```python
from build123d import *

# Parameters (mm, degrees)
F1_DEPTH      = 2
F2_DEPTH      = 42
F5_DEPTH      = 2
F7_DEPTH      = 2
F8_W          = 28.9586056024
F8_H          = 21
F9_DEPTH      = 25
F10_W         = 38.9921951145
F10_H         = 12
F11_DEPTH     = 2
F12_T1_DEPTH  = 12
F12_T6_DEPTH  = 51.7431402671
F12_T11_DEPTH = 51.7431402671
F12_T17_DEPTH = 40
F12_T22_DEPTH = 51.7431402671
F13_R         = 5


# Not quite as in the source:
# - a fillet or chamfer that OpenCascade refuses, or shapes differently, is made with other operations: its cross-section is extruded or revolved along the edge and cut away or added


with BuildPart() as f1:
    # F0 (on Top) → F1 (new body)
    with BuildSketch(Plane.XY):
        Polygon((16.9007111498, 56.5512960928), (-61.0992888502, 51.6762960928), (-61.0992888502, 18.6762960928), (16.9007111498, 13.8012960928), (18.9007111498, 13.6762960928), (18.9007111498, 15.6801985355), (16.9007111498, 15.8051985355), (-59.0992888502, 20.5551985355), (-59.0992888502, 49.79739365), (16.9007111498, 54.54739365), (18.9007111498, 54.67239365), (18.9007111498, 56.6762960928), align=None)
        Polygon((18.9007111498, 15.6801985355), (18.9007111498, 54.67239365), (16.9007111498, 54.54739365), (16.9007111498, 15.8051985355), align=None)
        Polygon((16.9007111498, 15.8051985355), (16.9007111498, 54.54739365), (-59.0992888502, 49.79739365), (-59.0992888502, 20.5551985355), align=None)
    extrude(amount=F1_DEPTH)

    # F0 (on Top) → F2 (join)
    with BuildSketch(Plane.XY):
        Polygon((16.9007111498, 56.5512960928), (-61.0992888502, 51.6762960928), (-61.0992888502, 18.6762960928), (16.9007111498, 13.8012960928), (18.9007111498, 13.6762960928), (18.9007111498, 15.6801985355), (16.9007111498, 15.8051985355), (-59.0992888502, 20.5551985355), (-59.0992888502, 49.79739365), (16.9007111498, 54.54739365), (18.9007111498, 54.67239365), (18.9007111498, 56.6762960928), align=None)
    extrude(amount=F2_DEPTH)

    # F3 (on face) → F5 (join)
    with BuildSketch(Plane(origin=(0.9249861815, 14.7997789033, 0), x_dir=(0.9980525785, -0.0623782862, 0), z_dir=(-0.0623782862, -0.9980525785, 0))):
        Polygon((18.3653086424, 55), (-62.1452981224, 42), (18.010799587, 42), align=None)
    extrude(amount=-F5_DEPTH)

    # F6 (on face) → F7 (join)
    with BuildSketch(Plane(origin=(-3.4549417367, 55.2790677874, 0), x_dir=(-0.9980525785, -0.0623782862, 0), z_dir=(-0.0623782862, 0.9980525785, 0))):
        Polygon((-22.3992737141, 55), (-22.3992737141, 42), (57.7568239953, 42), align=None)
    extrude(amount=-F7_DEPTH)

    # F8 (on face) → F9 (cut)
    with BuildSketch(Plane(origin=(-61.0992888502, 0, 0), x_dir=(0, -1, 0), z_dir=(-1, 0, 0))):
        with Locations((-35.0762708113, 31.5)):
            Rectangle(F8_W, F8_H)
    extrude(amount=-F9_DEPTH, mode=Mode.SUBTRACT)

    # F10 (on face) → F11 (join)
    with BuildSketch(Plane.YZ.offset(18.9007111498)):
        with Locations((35.1762960928, 21)):
            Rectangle(F10_W, F10_H)
    extrude(amount=-F11_DEPTH)

    # F12: fillet of radius 5 on 4 edges, made by hand

    # F12_s2 → F12_t1 (join)
    with BuildSketch(Plane.XY.offset(15)):
        with BuildLine():
            ThreePointArc((11.588819719, 16.1371917499), (15.324199345, 17.4833184516), (16.9007111498, 21.1274546423))
            Line((16.9007111498, 21.1274546423), (16.9007111498, 15.8051985355))
            Line((16.9007111498, 15.8051985355), (11.588819719, 16.1371917499))
        make_face()
        with BuildLine():
            ThreePointArc((11.588819719, 54.2154004356), (15.324199345, 52.869273734), (16.9007111498, 49.2251375432))
            Line((16.9007111498, 49.2251375432), (16.9007111498, 54.54739365))
            Line((16.9007111498, 54.54739365), (11.588819719, 54.2154004356))
        make_face()
    extrude(amount=F12_T1_DEPTH)


with BuildPart() as f12_tool4:
    # F12_s5 → F12_t6 (new body)
    with BuildSketch(Plane.XY.offset(2)):
        with BuildLine():
            ThreePointArc((-54.411180281, 20.2621917499), (-57.743425041, 21.8289664471), (-59.0992888502, 25.2524546423))
            Line((-59.0992888502, 25.2524546423), (-59.0992888502, 20.5551985355))
            Line((-59.0992888502, 20.5551985355), (-54.411180281, 20.2621917499))
        make_face()
    extrude(amount=F12_T6_DEPTH)

    split(bisect_by=Plane.XY.offset(21), keep=Keep.BOTTOM)


with BuildPart() as f1_1:
    add(f1.part)

    # F12_t3: union F12_tool4
    add(f12_tool4.part)


with BuildPart() as f12_tool9:
    # F12_s10 → F12_t11 (new body)
    with BuildSketch(Plane.XY.offset(-9.7431402671)):
        with BuildLine():
            ThreePointArc((-54.411180281, 20.2621917499), (-57.743425041, 21.8289664471), (-59.0992888502, 25.2524546423))
            Line((-59.0992888502, 25.2524546423), (-59.0992888502, 20.5551985355))
            Line((-59.0992888502, 20.5551985355), (-54.411180281, 20.2621917499))
        make_face()
    extrude(amount=F12_T11_DEPTH)

    split(bisect_by=Plane.XZ.offset(-20.5969680101), keep=Keep.TOP)

    split(bisect_by=Plane.XY.offset(21), keep=Keep.TOP)


with BuildPart() as f1_2:
    add(f1_1.part)

    # F12_t8: union F12_tool9
    add(f12_tool9.part)


with BuildPart() as f12_tool15:
    # F12_s16 → F12_t17 (new body)
    with BuildSketch(Plane.XY.offset(2)):
        with BuildLine():
            ThreePointArc((-54.411180281, 50.0904004356), (-57.743425041, 48.5236257384), (-59.0992888502, 45.1001375432))
            Line((-59.0992888502, 45.1001375432), (-59.0992888502, 49.79739365))
            Line((-59.0992888502, 49.79739365), (-54.411180281, 50.0904004356))
        make_face()
    extrude(amount=F12_T17_DEPTH)

    split(bisect_by=Plane.XZ.offset(-49.5555736125), keep=Keep.BOTTOM)


with BuildPart() as f1_3:
    add(f1_2.part)

    # F12_t14: union F12_tool15
    add(f12_tool15.part)


with BuildPart() as f12_tool20:
    # F12_s21 → F12_t22 (new body)
    with BuildSketch(Plane.XY.offset(2)):
        with BuildLine():
            ThreePointArc((-54.411180281, 50.0904004356), (-57.743425041, 48.5236257384), (-59.0992888502, 45.1001375432))
            Line((-59.0992888502, 45.1001375432), (-59.0992888502, 49.79739365))
            Line((-59.0992888502, 49.79739365), (-54.411180281, 50.0904004356))
        make_face()
    extrude(amount=F12_T22_DEPTH)

    split(bisect_by=Plane.XY.offset(21), keep=Keep.BOTTOM)


with BuildPart() as f1_4:
    add(f1_3.part)

    # F12_t19: union F12_tool20
    add(f12_tool20.part)

    # F13
    f13_edges = [f1_4.edges().sort_by_distance(p)[0] for p in [
        (18.963089, 55.678244, 55),
        (19.316908, 14.652235, 55),
    ]]
    fillet(f13_edges, radius=F13_R)


solid = f1_4.part
```
Part model, mm, in its own coordinate system. A direction names the side the tool comes from. Give positions to 0.01 mm unless a question says otherwise; leave off trailing zeros. Order: outer loops, then holes, each group sorted by start corner. A loop starts at its lowest first (then second) coordinate and runs counter-clockwise, first axis right, second up. Notation, with made-up numbers: M 19.25,53 L 75.25,53 A19 ccw 75.25,85 Z; hole C 66,8 d2. An arc over 180 degrees is marked long. Use a Markdown table: item, result. Add a question column.
(1) Drop flat-ended pins along their axis: P1, Ø1.7, axis at x = -58, y = 51, coming from the +Z side; P2, Ø21, axis at y = 39.5, z = 14.5, coming from the +X side; P3, Ø8, axis at x = -16.5, y = 36.5, coming from the +Z side; P4, Ø6, axis at x = -32.5, y = 33, coming from the -Z side. Give the stop position or say it passes through.
(2) Saw through at C-C, the plane z = 11.5. Give the cut face in (x, y), and give its area (3 significant figures).
(3) Saw through at B-B, the plane y = 31.5. Give the cut face in (x, z).
(4) Probe line 1 along Z through (x, y) = (8.5, 48); line 2 along Y through (x, z) = (-49.5, 35.5); line 3 along Y through (x, z) = (-51.5, 40). List the from-to ranges inside material, lowest first. Write a range as [from, to].
(5) Saw through at D-D, the plane x = -0.5. Give the cut face in (y, z), and give its area (3 significant figures).
(6) 3-axis set-ups, long thin cutter, end or side, ignore diameter. For faces 1 (the face through (18, 34, 15)), 2 (the face through (-59.099, 35, 11)), 3 (the face through (-59, 20.597, 32)), 4 (the face through (18, 34, 27)): which of +Z, -Z, +X, -X, +Y, -Y reach the whole face in a straight line?
(7) Saw through at A-A, the plane z = 28.5. Give the cut face in (x, y).
(8) Mould opens along Y. For faces 5 (the face through (-61.099, 35, 11)), 6 (the face through (-57.1, 49.1, 17.3)), 7 (the face through (18.962, 55.692, 45.612)) say: +Y half, -Y half, draft (parallel to the pull), parting line (faces both ways), or undercut.
Answer key:
| question | item | result |
|---|---|---|
| 1 | P1 | z = 42.63 |
| 1 | P2 | x = 18.9 |
| 1 | P3 | z = 2 |
| 1 | P4 | z = 0 |
| 2 | outline | M -61.1,18.68 L 18.9,13.68 L 18.9,15.68 L -54.41,20.26 A5 cw -59.1,25.25 L -59.1,45.1 A5 cw -54.41,50.09 L 18.9,54.67 L 18.9,56.68 L -61.1,51.68 Z |
| 2 | area | 388 mm^2 |
| 3 | outline | M -61.1,0 L 18.9,0 L 18.9,2 L -59.1,2 L -59.1,21 L -61.1,21 Z; M 16.9,15 L 18.9,15 L 18.9,27 L 16.9,27 Z |
| 4 | line 1 | [0, 2] |
| 4 | line 2 | [17.95, 19.96], [50.4, 52.4] |
| 4 | line 3 | [18.08, 20.08], [50.27, 52.28] |
| 5 | outline | M 14.89,0 L 55.46,0 L 55.46,51.85 L 53.46,51.83 L 53.46,2 L 16.89,2 L 16.89,51.78 L 14.89,51.8 Z |
| 5 | area | 281 mm^2 |
| 6 | face 1 | +X |
| 6 | face 2 | +Z |
| 6 | face 3 | -X |
| 6 | face 4 | +Z, +X |
| 7 | outline | M -61.1,18.68 L 18.9,13.68 L 18.9,15.68 L -54.41,20.26 A5 cw -55.92,20.6 L -61.1,20.6 Z; M -61.1,49.56 L -56.37,49.56 A5 cw -54.41,50.09 L 18.9,54.67 L 18.9,56.68 L -61.1,51.68 Z |
| 8 | face 5 | draft |
| 8 | face 6 | undercut |
| 8 | face 7 | +Y half |
